from build123d import *

# Parameters (mm, degrees)
F1_DEPTH = 76.2
F3_DEPTH = 101.6


with BuildPart() as f1:
    # F0 (on Front) → F1 (new body)
    with BuildSketch(Plane.XZ):
        Polygon((-15.662028, 37.975211), (-57.724428, 37.975211), (-71.931587, -33.654443), (-29.869187, -33.654443), align=None)
    extrude(amount=F1_DEPTH)

    # F2 (on Front) → F3 (cut, symmetric)
    with BuildSketch(Plane.XZ):
        Polygon((-32.971758, -30.479443), (-20.326851, 34.800211), (-54.859936, 34.800211), (-68.170242, -30.479443), align=None)
    extrude(amount=F3_DEPTH, both=True, mode=Mode.SUBTRACT)


solid = f1.part
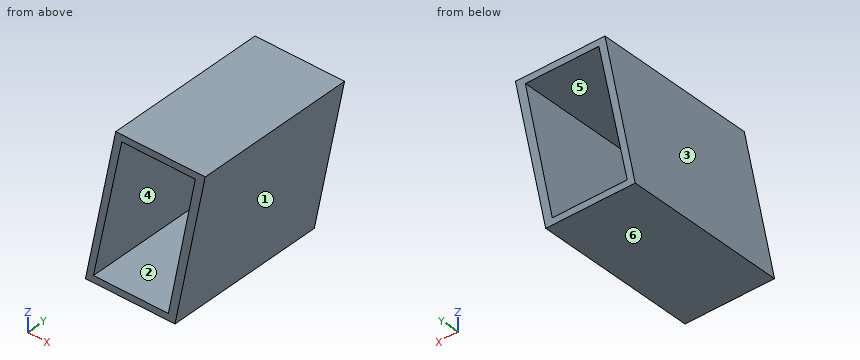
Can you work these out from the model? Positions are in its coordinate system, mm. Face numbers are marked on the shaded views. A direction names the side the tool comes from. Round coordinates to 2 decimals unless told otherwise and drop trailing zeros. Loops run counter-clockwise (first coordinate to the right, second up) from the corner with the lowest first, then second, coordinate; pieces in that order, holes last. Notation, with made-up numbers: (51.5, 33) - (57.5, 33) arc R19 cw to (57.5, 38) - close; hole circle Ø1 at (89, 38). An arc over 180 degrees is marked (long way). Write item = value, one per line. Start each with the question number.
(1) If I drill on probe 1 along Z at (x, y) = (-34, -30.5); probe 2 along X at (y, z) = (-63.5, -26); probe 3 along X at (y, z) = (-47, 25), over which ranges is the centre line in solid material (lowest first)? Write a range as [from, to].
(2) If we section it at A-A (x = -52): Please give me the cut outline in (y, z), and give its area (3 significant figures).
(3) For P1, Ø8, axis at y = -11, z = 19, coming from the -X side; P2, Ø2, axis at y = -63.5, z = -15.5, coming from the +X side; P3, Ø8, axis at y = -52.5, z = -16.5, coming from the -X side, each with a flat end and sliding along its axis, tell me the tip position at first contact or that it passes through.
(4) If we section it at B-B (z = 17.5): Please give me the cut outline in (x, y).
(5) If we section it at C-C (y = -46.5): Please give me the cut outline in (x, z), and give its area (3 significant figures).
(6) For the marked faces 1 and 2, which set-ups out of +Z, -Z, +X, -X, +Y, -Y let a thin tool reach every point of the face, with its end or its side?
(7) If we mould it in two halves opening along Z, with no side actions, what happens to the marked faces 3, 4, 5 and 6? For each: released by +Z, released by -Z, zero draft, split by the parting line, or undercut.
Ans:
q1.probe_1 = [-33.65, -30.48], [34.8, 37.98]
q1.probe_2 = [-70.41, -67.26], [-32.1, -28.35]
q1.probe_3 = [-60.3, -56.86], [-22.23, -18.24]
q2.outline = (-76.2, -33.65) - (0, -33.65) - (0, -30.48) - (-76.2, -30.48) - close; (-76.2, 34.8) - (0, 34.8) - (0, 37.98) - (-76.2, 37.98) - close
q2.area = 484 mm²
q3.P1 = -62.28
q3.P2 = -26.07
q3.P3 = -69.32
q4.outline = (-61.79, -76.2) - (-58.39, -76.2) - (-58.39, 0) - (-61.79, 0) - close; (-23.68, -76.2) - (-19.72, -76.2) - (-19.72, 0) - (-23.68, 0) - close
q5.outline = (-71.93, -33.65) - (-29.87, -33.65) - (-15.66, 37.98) - (-57.72, 37.98) - close; hole (-68.17, -30.48) - (-32.97, -30.48) - (-20.33, 34.8) - (-54.86, 34.8) - close
q5.area = 737 mm²
q6.face_1 = -Z, +X, +Y, -Y
q6.face_2 = +Y, -Y
q7.face_3 = released by +Z
q7.face_4 = undercut
q7.face_5 = undercut
q7.face_6 = released by -Z
